Input: part model. Units: mm. Frame: model coordinates. Round coordinates to 2 decimals unless told otherwise and drop trailing zeros. Loops run counter-clockwise (first coordinate to the right, second up) from the corner with the lowest first, then second, coordinate; pieces in that order, holes last. Notation, with made-up numbers: (70.25, 42.25) - (76.25, 42.25) arc R22 ccw to (76.25, 78.25) - close; hole circle Ø5 at (-38.5, 26). An arc over 180 degrees is marked (long way). Use CSV: the item, a comma, the result in double quotes. Start each with the question number.
1. Cut plane C-C (x = 8.5). Return loops of the section in (y, z) (3 decimals).
2. Cut plane D-D (y = 4.5). Return loops of the section in (x, z) (3 decimals), and give its area (3 significant figures).
3. Cut plane A-A (x = -1.5). Return loops of the section in (y, z) (3 decimals), and give its area (3 significant figures).
4. Pin query (flat end, axial travel): P1, Ø5, axis at y = -6, z = -3.5, coming from the -X side; P2, Ø6, axis at y = -10, z = -1.5, coming from the +X side; P3, Ø8, axis at y = 1, z = 17, coming from the +X side. Return the tip coordinate at first contact, or that it passes through.
5. Material intervals for probe 1 along Z at (x, y) = (22, 1.75) (3 decimals); probe 2 along X at (y, z) = (-3.5, 18); probe 3 along X at (y, z) = (-2, -3), sorted ascending. Write a range as from..to.
6. Pull-direction query (X, two-part tool) for faces 1 (the flat face through (9, 0, -9.525)), 2 (the flat face through (25.49, -6.26, 0.13)), 3 (the cylindrical face through (-1.38, -6.2, 7.69)); classes: +X half, -X half, draft (parallel to the pull), parting line (faces both ways), or undercut.
7. Cut plane B-B (y = -4). Return loops of the section in (x, z) (3 decimals), and give its area (3 significant figures).
```python
from build123d import *

# Parameters (mm, degrees)
F0_R     = 6.35
F1_DEPTH = 25.4
F2_DEPTH = 9.525
F4_DEPTH = 12.7


with BuildPart() as f1:
    # F0 (on Top) → F1 (new body)
    with BuildSketch(Plane.XY):
        with BuildLine():
            ThreePointArc((0, -12.7), (8.980256, -8.980256), (12.7, 0))
            ThreePointArc((12.7, 0), (8.980256, 8.980256), (0, 12.7))
            ThreePointArc((0, 12.7), (-12.7, 0), (0, -12.7))
        make_face()
        Circle(F0_R, mode=Mode.SUBTRACT)
    extrude(amount=F1_DEPTH)

    # F0 (on Top) → F2 (join, symmetric)
    with BuildSketch(Plane.XY):
        with BuildLine():
            ThreePointArc((0, -12.7), (8.980256, -8.980256), (12.7, 0))
            ThreePointArc((12.7, 0), (8.980256, 8.980256), (0, 12.7))
            ThreePointArc((0, 12.7), (-12.7, 0), (0, -12.7))
        make_face()
        Circle(F0_R, mode=Mode.SUBTRACT)
        with BuildLine():
            ThreePointArc((0, 12.7), (8.980256, 8.980256), (12.7, 0))
            ThreePointArc((12.7, 0), (8.980256, -8.980256), (0, -12.7))
            Line((0, -12.7), (31.75, -12.7))
            Line((31.75, -12.7), (31.75, 12.7))
            Line((31.75, 12.7), (0, 12.7))
        make_face()
    extrude(amount=F2_DEPTH, both=True)

    # F3 (on Top) → F4 (cut, symmetric)
    with BuildSketch(Plane.XY):
        Polygon((31.75, 0), (19.05, -12.7), (31.75, -12.7), align=None)
    extrude(amount=F4_DEPTH, both=True, mode=Mode.SUBTRACT)


solid = f1.part
```
Established:
1,outline,"(-12.7, -9.525) - (12.7, -9.525) - (12.7, 9.525) - (9.436, 9.525) - (9.436, 25.4) - (-9.436, 25.4) - (-9.436, 9.525) - (-12.7, 9.525) - close"
2,outline,"(-11.876, -9.525) - (-4.48, -9.525) - (-4.48, 25.4) - (-11.876, 25.4) - close; (4.48, -9.525) - (31.75, -9.525) - (31.75, 9.525) - (11.876, 9.525) - (11.876, 25.4) - (4.48, 25.4) - close"
2,area,"895 mm2"
3,outline,"(-12.611, -9.525) - (-6.17, -9.525) - (-6.17, 25.4) - (-12.611, 25.4) - close; (6.17, -9.525) - (12.611, -9.525) - (12.611, 25.4) - (6.17, 25.4) - close"
3,area,"450 mm2"
4,P1,"stops at x = -12.21"
4,P2,"stops at x = 24.75"
4,P3,"stops at x = 12.7"
5,probe 1,"z = -9.525..9.525"
5,probe 2,"x = -12.21..-5.3, 5.3..12.21"
5,probe 3,"x = -12.54..-6.03, 6.03..29.75"
6,face 1,"draft"
6,face 2,"+X half"
6,face 3,"undercut"
7,outline,"(-12.054, -9.525) - (-4.932, -9.525) - (-4.932, 25.4) - (-12.054, 25.4) - close; (4.932, -9.525) - (27.75, -9.525) - (27.75, 9.525) - (12.054, 9.525) - (12.054, 25.4) - (4.932, 25.4) - close"
7,area,"796 mm2"
